Input: part model. Units: mm. Frame: model coordinates. A direction names the side the tool comes from. Coordinates: 2 decimals unless noted, no trailing zeros. Loops run counter-clockwise (first coordinate to the right, second up) from the corner with the lowest first, then second, coordinate; pieces in that order, holes last.
Autodesk Inventor part; units mm, degrees
ref_plane "YZ Plane" through (0, 0, 0) normal (1, 0, 0) x (0, 1, 0)
ref_plane "XZ Plane" through (0, 0, 0) normal (0, 1, 0) x (-1, 0, 0)
ref_plane "XY Plane" through (0, 0, 0) normal (0, 0, 1) x (1, 0, 0)
sketch "Esquisse1" plane through (0, 0, 0) normal (0, 1, 0) x (-1, 0, 0)
  arc A0 (51.3642, -31.0232) -> (51.3642, 31) centre (0, -0.0116) ccw
  arc A1 (129, -9.7584) -> (129, 9.7352) centre (136, -0.0116) ccw
  arc A2 (51.3642, 31) -> (129, 9.7352) centre (116, 114.6263) ccw
  line L0 (64, -0.0116) -> (129, -0.0116) construction
  arc A3 (129, -9.7584) -> (129, 9.7352) centre (136, -0.0116) ccw
  arc A4 (129, -9.7584) -> (51.3642, -31.0232) centre (116, -114.6495) ccw
  circle A5 centre (136, -0.0116) radius 11
  point P0 (0, 0)
  dimension "d0" = 120
  dimension "d1" = 24
  dimension "d2" = 22
extrude "Extrusion1" add sketch "Esquisse1" along normal blind 10
ref_plane "Plan de construction1" through (-51.3642, 0, -31.0232) normal (1, 0, 0) x (0, 1, 0)
sketch "Esquisse2" plane through (-51.3642, 0, -31.0232) normal (1, 0, 0) x (0, 1, 0)
  line L0 (5, 64.5652) -> (5, -0.1304) construction
  line L1 (3, 49) -> (7, 49)
  line L2 (8, 47.6173) -> (8, 44)
  line L3 (2, 44) -> (2, 47.6173)
  line L4 (2, 49) -> (8, 43) construction
  line L5 (8, 49) -> (2, 43) construction
  line L6 (8, 18) -> (8, 14.5151)
  line L7 (7, 13) -> (3, 13)
  line L8 (2, 14.5151) -> (2, 18)
  line L9 (2, 19) -> (8, 13) construction
  line L10 (8, 19) -> (2, 13) construction
  line L11 (10, 62.0232) -> (10, 0)
  line L12 (0, 0) -> (10, 0)
  line L13 (0, 62.0232) -> (10, 62.0232)
  spline S0 degree 4 poles (7.6671, 44) (6.4354, 47.4326) (4.9707, 48.7302) (3.6119, 47.2748) (2.3584, 44) knots 0 0 0 0 0 1 1 1 1 1
  spline S1 degree 4 poles (7.6511, 18) (6.3929, 14.6165) (5, 13.0055) (3.6071, 14.6165) (2.3489, 18) knots 0 0 0 0 0 1 1 1 1 1
  arc A0 (8, 47.4506) -> (7, 49) centre (6.4288, 47.5339) ccw
  arc A1 (3, 49) -> (2, 47.4506) centre (3.5712, 47.5339) ccw
  arc A2 (7, 13) -> (8, 14.5151) centre (6.3523, 14.5151) ccw
  arc A3 (2, 14.5151) -> (3, 13) centre (3.6477, 14.5151) ccw
  line L14 (2, 18) -> (2.3489, 18)
  line L15 (7.6511, 18) -> (8, 18)
  line L16 (2.776, 16.8516) -> (1.9218, 19.1484) construction
  arc A4 (2.0268, 18.9251) -> (2.7095, 17.0892) centre (24.2353, 26.1386) ccw construction
  line L17 (8.0782, 19.1484) -> (7.224, 16.8516) construction
  arc A5 (7.2905, 17.0892) -> (7.9732, 18.9251) centre (-14.2353, 26.1386) ccw construction
  line L18 (2, 44) -> (2.3584, 44)
  line L19 (7.6671, 44) -> (8, 44)
  line L20 (2.7888, 45.1243) -> (1.9281, 42.8757) construction
  arc A6 (2.7221, 44.891) -> (2.0343, 43.0939) centre (22.8073, 36.1728) ccw construction
  line L21 (8.0877, 42.828) -> (7.2466, 45.172) construction
  arc A7 (7.9784, 43.0548) -> (7.3065, 44.9274) centre (-10.0817, 37.6313) ccw construction
  point P0 (0, 31.0232)
  point P1 (5, 46)
  point P2 (5, 16)
  dimension "d10" = 2
  dimension "d11" = 2
  dimension "d12" = 13
  dimension "d13" = 13.0232
  dimension "d19" = 1
  dimension "d20" = 1
  dimension "d21" = 1
  dimension "d22" = 1
extrude "Extrusion2" add sketch "Esquisse2" against normal blind 10
sketch "Esquisse3" plane through (-51.3642, 8, 16.594) normal (0, 1, 0) x (1, 0, 0)
  point P0 (51.3642, 16.594)
sketch "Esquisse4" plane through (-51.3642, 8, 16.594) normal (0, 1, 0) x (1, 0, 0)
  point P0 (51.3642, 16.594)
ref_plane "Plan de construction7" through (-55.0062, 0, -31.0232) normal (1, 0, 0) x (0, 1, 0)
ref_plane "Plan de construction6" through (-60.1142, 0, -31.0232) normal (1, 0, 0) x (0, 1, 0)
fillet "Congé2" radius 1 1 edges at (-60, 0, -0.0116)
sketch "Esquisse7" plane through (-51.3642, 0, -31.0232) normal (1, 0, 0) x (0, 1, 0)
  line L0 (7, 49) -> (3, 49)
  line L1 (4, 49) -> (6, 49)
  line L2 (6, 49) -> (6, 50)
  line L3 (6, 50) -> (4, 50)
  line L4 (4, 50) -> (4, 49)
  line L5 (3, 13) -> (7, 13)
  line L6 (4, 13) -> (6, 13)
  line L7 (6, 13) -> (6, 12)
  line L8 (6, 12) -> (4, 12)
  line L9 (4, 12) -> (4, 13)
  point P0 (0, 31.0232)
extrude "Extrusion5" add sketch "Esquisse7" against normal blind 1
ref_plane "Plan de construction8" through (-51.3642, 4, -19.0232) normal (0, -1, 0) x (1, 0, 0)
sketch "Esquisse8" plane through (-51.3642, 4, -19.0232) normal (0, -1, 0) x (1, 0, 0)
  line L0 (-1, 37) -> (-1, 38)
  line L1 (0, 37) -> (-1, 37)
  line L2 (0, 1) -> (0, 0)
  line L3 (-1, 1) -> (-1, 0)
  line L4 (0, 1) -> (-5.8685, 1)
  line L5 (0, 38) -> (-1, 38)
  line L6 (-1, 37) -> (-1, 38)
  line L7 (-1, 0) -> (-1, 1)
  line L8 (0, 0) -> (0, 1)
  line L9 (-1, 1) -> (0, 1)
  line L10 (-1, 0) -> (-1, 1)
  line L11 (0, 0) -> (-1, 0)
  line L12 (0, 0) -> (0, 1)
  line L13 (-1, 1) -> (0, 1)
  line L14 (-1, 0) -> (-1, 1)
  line L15 (0, 0) -> (-1, 0)
  line L16 (0, 38) -> (0, 37)
  line L17 (0, 38) -> (-1, 38)
  line L18 (-1, 37) -> (-1, 38)
  line L19 (0, 37) -> (-1, 37)
  line L20 (0, 0) -> (-1, 0)
  line L21 (0, 1) -> (-1, 1)
  arc A0 (-0.1986, 0) -> (-1, 1) centre (-1.3637, -0.1126) ccw
  line L22 (0, 38) -> (-1, 38)
  arc A1 (-1, 37) -> (-0.1986, 38) centre (-1.3356, 38.0901) ccw
  point P0 (51.3642, 19.0232)
extrude "Extrusion6" cut sketch "Esquisse8" against normal blind 3.25 contours L0 L5 A1 | A0 L11 L3
sketch "Esquisse9" plane through (0, 0, 0) normal (0, 1, 0) x (-1, 0, 0)
  line L0 (51.3642, 17.9768) -> (57.24, 17.9768)
  circle A0 centre (0, 0) radius 54.4192
extrude "Extrusion7" cut sketch "Esquisse9" along normal blind 10.25
sketch "Esquisse10" plane through (0, 0, 0) normal (0, -1, 0) x (1, 0, 0)
  arc A0 (-53.4086, 29.459) -> (-53.4086, -29.4822) centre (0, -0.0116) ccw
  arc A1 (-129, 9.7352) -> (-53.4086, 29.459) centre (-116, 114.6263) ccw
  arc A2 (-129, 9.7352) -> (-129, -9.7584) centre (-136, -0.0116) ccw
  arc A3 (-53.4086, -29.4822) -> (-129, -9.7584) centre (-116, -114.6495) ccw
  circle A4 centre (-136, -0.0116) radius 11
  arc A5 (-59.6325, 22.1419) -> (-59.6325, -22.1651) centre (0, -0.0116) ccw
  arc A6 (-124.8494, 6.6802) -> (-59.6325, 22.1419) centre (-116, 114.6263) ccw
  arc A7 (-124.8494, -6.7035) -> (-124.8494, 6.6802) centre (-136, -0.0116) ccw
  arc A8 (-59.6325, -22.1651) -> (-124.8494, -6.7035) centre (-116, -114.6495) ccw
  point P0 (0, 0)
extrude "Extrusion8" cut sketch "Esquisse10" against normal blind 8 contours A5 A8 A7 A6
properties part number "Aile"
Item 1: Section query B-B (x = -120.5). Output: boundary loops of the cut face in (y, z).
Result:
outline: (0, -9.05) - (10, -9.05) - (10, 9.03) - (0, 9.03) - (0, 6.41) - (8, 6.41) - (8, -6.43) - (0, -6.43) - close
Item 2: Line query: L1, parallel to Z at x = -136, y = 5; L2, parallel to Z at x = -92, y = 3.5; L3, parallel to X at y = 3.5, z = 1.5. Output: solid intervals per line, ascending.
Result:
L1: z = -12.01 to -11.01, 10.99 to 11.99
L2: z = -11.72 to -9.03, 9.01 to 11.69
L3: x = -147.9 to -146.9, -125.1 to -123.08, -63.6 to -59.98
Item 3: Mould query, pull axis X, two halves, no side actions, for faces 5 (the face through (-55, 8, -15)), 6 (the face through (-91.48, 3.94, 9.13)), 7 (the face through (-51.83, 4.29, -16.58)), 8 (the face through (-88.636, 4.93, 12.536)). Classes: +X half, -X half, draft (parallel to the pull), parting line (faces both ways), or undercut.
Result:
face 5: draft
face 6: undercut
face 7: +X half
face 8: undercut
Item 4: Contact query for flat-ended pins moving along their axis: P1, Ø6, axis at y = 7.5, z = 24, coming from the +X side; P2, Ø0.8, axis at x = -51.5, z = -18.5, coming from the +Y side; P3, Ø2, axis at x = -137.5, y = 1, coming from the -Z side. Output: stop coordinate, or through.
Result:
P1: stops at x = -53.58
P2: stops at y = 6
P3: stops at z = -12
Item 5: Reachability of faces 1 (the face through (-51.814, 4.958, 16.637)), 2 (the face through (-55, 2, 15)), 3 (the face through (-148, 5, 0)), 4 (the face through (-55, 8, 15)) from +Z, -Z, +X, -X, +Y, -Y: full face, straight path, thin tool, end or side. Return the list, or none.
Result:
face 1: +X, +Y, -Y
face 2: +X, -Y
face 3: +Y, -Y
face 4: +X, +Y
Item 6: Section query A-A (x = -136). Output: boundary loops of the cut face in (y, z), then the cut area to 3 significant figures.
Result:
outline: (0, -12.01) - (10, -12.01) - (10, -11.01) - (0, -11.01) - close; (0, 10.99) - (10, 10.99) - (10, 11.99) - (0, 11.99) - close
area: 20.0 mm2
Item 7: Section query C-C (x = -98). Output: boundary loops of the cut face in (y, z).
Result:
outline: (0, -10.5) - (10, -10.5) - (10, 10.48) - (0, 10.48) - (0, 7.82) - (8, 7.82) - (8, -7.85) - (0, -7.85) - close
